Build history of the part. All positions in model axes, mm. Face numbers are marked on the shaded views. A direction names the side the tool comes from. Round coordinates to 2 decimals unless told otherwise and drop trailing zeros. Write each loop counter-clockwise with the first axis right and the second up, starting at its lowest first coordinate (ties: lowest second). Pieces come first, ordered by that corner, then holes.
from build123d import *

# Parameters (mm, degrees)
SKETCH1_R           = 1.7
BOSS_EXTRUDE1_DEPTH = 11
SKETCH2_W           = 10
SKETCH2_H           = 7
CUT_EXTRUDE1_DEPTH  = 1.5


with BuildPart() as part:
    # Sketch1 → Boss-Extrude1 (new body)
    with BuildSketch(Plane.XY):
        with BuildLine():
            Line((-5, -8), (-5, 8))
            ThreePointArc((-5, 8), (0, 13), (5, 8))
            Line((5, 8), (5, -8))
            ThreePointArc((5, -8), (0, -13), (-5, -8))
        make_face()
        with Locations((0, 8)):
            Circle(SKETCH1_R, mode=Mode.SUBTRACT)
        with Locations((0, -8)):
            Circle(SKETCH1_R, mode=Mode.SUBTRACT)
    extrude(amount=BOSS_EXTRUDE1_DEPTH)

    # Sketch2 → Cut-Extrude1 (cut)
    with BuildSketch(Plane.XY.offset(11)):
        Rectangle(SKETCH2_W, SKETCH2_H)
    extrude(amount=-CUT_EXTRUDE1_DEPTH, mode=Mode.SUBTRACT)


solid = part.part
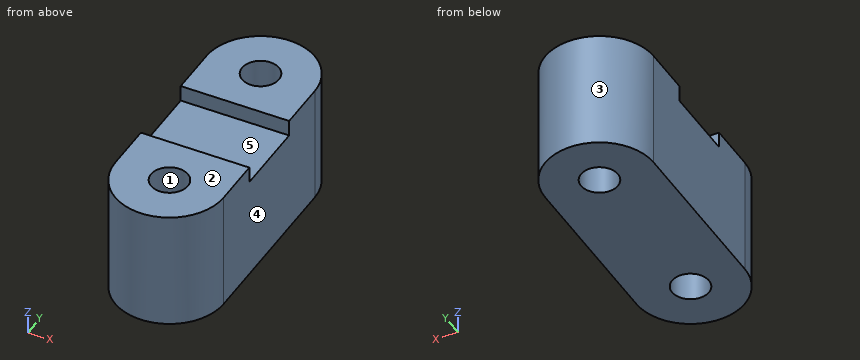
1) Pin check, flat tips, straight feed: pin 1 Ø4 at (x, y) = (0, -8) entering from -Z; pin 2 Ø2.5 at (x, y) = (0, 8) entering from +Z; pin 3 Ø1.5 at (x, z) = (-1, 10) entering from -Y; pin 4 Ø1 at (y, z) = (-9.5, 3) entering from +X. Stop position of each tip, or through.
Results:
pin 1: stops at z = 0
pin 2: passes through
pin 3: stops at y = -12.99
pin 4: stops at x = 4.9
2) Slice it at B-B (z = 8.5). Write the cut outline in (x, y), plus the area to 3 significant figures.
Results:
outline: (-5, -8) arc R5 ccw to (5, -8) - (5, 8) arc R5 ccw to (-5, 8) - close; hole circle Ø3.4 at (0, -8); hole circle Ø3.4 at (0, 8)
area: 220 mm2
3) Which spindle directions (+Z, -Z, +X, -X, +Y, -Y) get a long thin tool onto all of the face, cutting with end or side? Do the marked faces 4 and 5. Say none if no direction does.
Results:
face 4: +Z, -Z, +X, +Y, -Y
face 5: +Z, +X, -X
4) Slice it at A-A (x = 0). Write the cut outline in (y, z), plus the area to 3 significant figures.
Results:
outline: (-13, 0) - (-9.7, 0) - (-9.7, 11) - (-13, 11) - close; (-6.3, 0) - (6.3, 0) - (6.3, 11) - (3.5, 11) - (3.5, 9.5) - (-3.5, 9.5) - (-3.5, 11) - (-6.3, 11) - close; (9.7, 0) - (13, 0) - (13, 11) - (9.7, 11) - close
area: 201 mm2
5) Mould opens along Y. For the marked faces 1, 2 and 3 say: released by +Y, released by -Y, zero draft, split by the parting line, or undercut.
Results:
face 1: undercut
face 2: zero draft
face 3: released by +Y
6) Wall check: L1, parallel to Y at x = 0, z = 2.5; L2, parallel to Y at x = -1, z = 5.5; L3, parallel to Y at x = 1, z = 9.75. Give the ranges that are in metal, low to high.
Results:
L1: y = -13 to -9.7, -6.3 to 6.3, 9.7 to 13
L2: y = -12.9 to -9.37, -6.63 to 6.63, 9.37 to 12.9
L3: y = -12.9 to -9.37, -6.63 to -3.5, 3.5 to 6.63, 9.37 to 12.9
7) Slice it at C-C (y = -9.25). Write the cut outline in (x, z).
Results:
outline: (-4.84, 0) - (-1.15, 0) - (-1.15, 11) - (-4.84, 11) - close; (1.15, 0) - (4.84, 0) - (4.84, 11) - (1.15, 11) - close
8) Slice it at D-D (x = -4.5). Write the cut outline in (y, z).
Results:
outline: (-10.18, 0) - (10.18, 0) - (10.18, 11) - (3.5, 11) - (3.5, 9.5) - (-3.5, 9.5) - (-3.5, 11) - (-10.18, 11) - close
